For this review, take the finished solid that the model builds, in its own axes (mm). Give positions to 0.01 mm unless a question says otherwise; leave off trailing zeros. Loops run counter-clockwise (first coordinate to the right, second up) from the corner with the lowest first, then second, coordinate; pieces in that order, holes last. Notation, with made-up numbers: M -9,53 L 38,53 A36 cw 38,91 Z; hole C 51.5,-13 d10. An arc over 180 degrees is marked long. Use CSV: the item, a comma, the result in double quotes. Start each with the question number.
1. Take a section at B-B, the plane y = 18.25. Write out the cut boundary in (x, z) (3 decimals), and give its area (3 significant figures).
2. To check wall thickness, follow line 1 (X direction, y = 13.5, z = 2.5); line 2 (X direction, y = 14, z = 0.85); line 3 (X direction, y = 5.5, z = 0.25). State the ranges of each line that lie inside material, in increasing order. Write a range as [from, to].
3. Take a section at A-A, the plane x = 16. Write out the cut boundary in (y, z) (3 decimals), and give its area (3 significant figures).
4. The part is to be moulded in two halves that separate along X. For faces 1 (the face through (70, 15, 2)), 2 (the face through (28.932, 9.638, 1.565)), 3 (the face through (42, 15, 3.175)), say which applies: pulls with the +X half, pulls with the -X half, needs draft (parallel to the pull), parting line crosses it, or undercut.
5. Insertion check: P1, Ø4, axis at x = 44.5, y = 20, coming from the -Z side. The pin has a flat end and moves straight along its axis. Give the tip position at first contact, or say it passes through.
6. Take a section at D-D, the plane x = 3. Write out the cut boundary in (y, z) (3 decimals).
7. Take a section at C-C, the plane z = 1.05. Write out the cut boundary in (x, y).
from build123d import *

# Parameters (mm, degrees)
SKETCH1_W             = 70
SKETCH1_H             = 30
SKETCH1_R             = 2.4892
SKETCH1_R_2           = 1.4986
SKETCH1_R_3           = 14
BOSS_EXTRUDE2_DEPTH   = 3.175
F_2_CLEARANCE_HOLE1_D = 2.4384


with BuildPart() as part:
    # Sketch1 → Boss-Extrude2 (new body)
    with BuildSketch(Plane.XY):
        with Locations((35, 15)):
            Rectangle(SKETCH1_W, SKETCH1_H)
        with Locations((55, 15)):
            Circle(SKETCH1_R, mode=Mode.SUBTRACT)
        with Locations((37.166699296, 13)):
            Circle(SKETCH1_R_2, mode=Mode.SUBTRACT)
        with Locations((16, 15)):
            Circle(SKETCH1_R_3, mode=Mode.SUBTRACT)
    extrude(amount=BOSS_EXTRUDE2_DEPTH)

    # #2 Clearance Hole1 (through all)
    with Locations(Plane.XY.offset(3.175)):
        with Locations((67, 3), (67, 27), (3, 27), (3, 3)):
            Hole(F_2_CLEARANCE_HOLE1_D / 2)


solid = part.part
Result set:
1,outline,"M 0,0 L 2.382,0 L 2.382,3.175 L 0,3.175 Z; M 29.618,0 L 70,0 L 70,3.175 L 29.618,3.175 Z"
1,area,"136 mm2"
2,line 1,"[0, 2.08], [29.92, 35.75], [38.58, 53.01], [56.99, 70]"
2,line 2,"[0, 2.04], [29.96, 36.05], [38.28, 52.72], [57.28, 70]"
2,line 3,"[0, 5.72], [26.28, 70]"
3,outline,"M 0,0 L 1,0 L 1,3.175 L 0,3.175 Z; M 29,0 L 30,0 L 30,3.175 L 29,3.175 Z"
3,area,"6.35 mm2"
4,face 1,"pulls with the +X half"
4,face 2,"undercut"
4,face 3,"needs draft"
5,P1,"z = 0"
6,outline,"M 0,0 L 1.781,0 L 1.781,3.175 L 0,3.175 Z; M 4.219,0 L 9.804,0 L 9.804,3.175 L 4.219,3.175 Z; M 20.196,0 L 25.781,0 L 25.781,3.175 L 20.196,3.175 Z; M 28.219,0 L 30,0 L 30,3.175 L 28.219,3.175 Z"
7,outline,"M 0,0 L 70,0 L 70,30 L 0,30 Z; hole C 3,3 d2.44; hole C 3,27 d2.44; hole C 16,15 d28; hole C 37.17,13 d3; hole C 55,15 d4.98; hole C 67,3 d2.44; hole C 67,27 d2.44"
